Part model, mm, in its own coordinate system. Face numbers are marked on the shaded views. A direction names the side the tool comes from. Give positions to 0.01 mm unless a question says otherwise; leave off trailing zeros. Order: outer loops, then holes, each group sorted by start corner. A loop starts at its lowest first (then second) coordinate and runs counter-clockwise, first axis right, second up. Notation, with made-up numbers: (12.25, -10) - (46.25, -10) arc R12 ccw to (46.25, 13) - close; hole circle Ø9 at (-28, -36). An arc over 180 degrees is marked (long way). One line per item, written item: value.
```python
from build123d import *

# Parameters (mm, degrees)
SKETCH1_R                = 19
BOSS_EXTRUDE1_DEPTH      = 3.5
SKETCH2_R                = 30
SKETCH2_R_2              = 19
SKETCH2_R_3              = 2.8
BOSS_EXTRUDE2_DEPTH      = 7
BOSS_EXTRUDE3_DEPTH      = 2
BOSS_EXTRUDE3_DEPTH_BACK = 7
SKETCH4_R                = 2.9
SKETCH5_R                = 5
BOSS_EXTRUDE4_DEPTH      = 3
CUT_EXTRUDE1_START       = -10
SKETCH3_R                = 19
CUT_EXTRUDE1_DEPTH       = 10
CUT_EXTRUDE3_START       = -13
CUT_EXTRUDE3_DEPTH       = 13
FILLET1_R                = 10
FILLET2_R                = 5
CUT_EXTRUDE4_START       = -4
SKETCH8_R                = 4
SKETCH8_R_2              = 19
CUT_EXTRUDE4_DEPTH       = 4
FILLET3_R                = 1


with BuildPart() as part:
    # Sketch1 → Boss-Extrude1 (new body)
    with BuildSketch(Plane(origin=(0, 0, 0), x_dir=(1, 0, 0), z_dir=(0, 1, 0))):
        with Locations(Location((0, 0, 0), (0, 0, 270))):
            Circle(SKETCH1_R)
    extrude(amount=BOSS_EXTRUDE1_DEPTH)

    # Sketch2 → Boss-Extrude2 (add)
    with BuildSketch(Plane(origin=(0, 0, 0), x_dir=(1, 0, 0), z_dir=(0, 1, 0))):
        with Locations(Location((0, 0, 0), (0, 0, 270))):
            Circle(SKETCH2_R)
        with Locations(Location((0, 0, 0), (0, 0, 270))):
            Circle(SKETCH2_R_2, mode=Mode.SUBTRACT)
        with Locations(Location((0, 25, 0), (0, 0, 270))):
            Circle(SKETCH2_R_3, mode=Mode.SUBTRACT)
        with Locations(Location((21.650635095, -12.5, 0), (0, 0, 270))):
            Circle(SKETCH2_R_3, mode=Mode.SUBTRACT)
        with Locations(Location((-21.650635095, -12.5, 0), (0, 0, 270))):
            Circle(SKETCH2_R_3, mode=Mode.SUBTRACT)
    extrude(amount=BOSS_EXTRUDE2_DEPTH)

    # Sketch4 → Boss-Extrude3 (add, two sides: drawn at the far end of the back side and taken through both)
    with BuildSketch(Plane.XZ.offset(-BOSS_EXTRUDE3_DEPTH_BACK)):
        with Locations(Location((-21.650635095, 12.5, 0), (0, 0, 270))):
            Circle(SKETCH4_R)
        with Locations(Location((21.650635095, 12.5, 0), (0, 0, 270))):
            Circle(SKETCH4_R)
        with Locations(Location((0, -25, 0), (0, 0, 270))):
            Circle(SKETCH4_R)
    extrude(amount=BOSS_EXTRUDE3_DEPTH + BOSS_EXTRUDE3_DEPTH_BACK)

    # Sketch5 → Boss-Extrude4 (add)
    with BuildSketch(Plane(origin=(0, 7, 0), x_dir=(1, 0, 0), z_dir=(0, 1, 0))):
        with Locations((-26.103110985, -14.7860609)):
            Circle(SKETCH5_R)
        with Locations((0.246451131, 29.99898768)):
            Circle(SKETCH5_R)
        with Locations((25.856659853, -15.212926781)):
            Circle(SKETCH5_R)
    extrude(amount=-BOSS_EXTRUDE4_DEPTH)

    # Sketch3 → Cut-Extrude1 (cut)
    with BuildSketch(Plane(origin=(0, 3.5, 0), x_dir=(1, 0, 0), z_dir=(0, 1, 0)).offset(CUT_EXTRUDE1_START)):
        with Locations(Location((0, 0, 0), (0, 0, 270))):
            Circle(SKETCH3_R)
    extrude(amount=CUT_EXTRUDE1_DEPTH, mode=Mode.SUBTRACT)

    # Sketch7 → Cut-Extrude3 (cut)
    with BuildSketch(Plane(origin=(0, 7, 0), x_dir=(1, 0, 0), z_dir=(0, 1, 0)).offset(CUT_EXTRUDE3_START)):
        with BuildLine():
            ThreePointArc((-29.54423259, -5.20944533), (-25.980762114, 15), (-10.2606043, 28.190778624))
            Line((-10.2606043, 28.190778624), (-13.773984089, 37.84371026))
            Line((-13.773984089, 37.84371026), (-43.939319858, -7.747687605))
            Line((-43.939319858, -7.747687605), (-29.54423259, -5.20944533))
        make_face()
        with BuildLine():
            ThreePointArc((-26.13264562, -4.6078905), (-22.980662881, 13.267891901), (-9.075772579, 24.935480225))
            Line((-9.075772579, 24.935480225), (-10.2606043, 28.190778624))
            ThreePointArc((-10.2606043, 28.190778624), (-25.980762114, 15), (-29.54423259, -5.20944533))
            Line((-29.54423259, -5.20944533), (-26.13264562, -4.6078905))
        make_face()
        with BuildLine():
            Line((15.259965643, 41.926411025), (10.2606043, 28.190778624))
            ThreePointArc((10.2606043, 28.190778624), (25.980762114, 15), (29.54423259, -5.20944533))
            Line((29.54423259, -5.20944533), (39.660606503, -6.993234998))
            Line((39.660606503, -6.993234998), (15.259965643, 41.926411025))
        make_face()
        with BuildLine():
            Line((10.2606043, 28.190778624), (9.075772579, 24.935480225))
            ThreePointArc((9.075772579, 24.935480225), (21.736841548, 15.220300308), (26.535783801, 0))
            ThreePointArc((26.535783801, 0), (26.434807132, -2.312745947), (26.13264562, -4.6078905))
            Line((26.13264562, -4.6078905), (29.54423259, -5.20944533))
            ThreePointArc((29.54423259, -5.20944533), (25.980762114, 15), (10.2606043, 28.190778624))
        make_face()
        with BuildLine():
            Line((28.679354216, -34.17872342), (19.283628291, -22.981333294))
            ThreePointArc((19.283628291, -22.981333294), (0, -30), (-19.283628291, -22.981333294))
            Line((-19.283628291, -22.981333294), (-25.886622414, -30.850475262))
            Line((-25.886622414, -30.850475262), (28.679354216, -34.17872342))
        make_face()
        with BuildLine():
            Line((19.283628291, -22.981333294), (17.056873041, -20.327589725))
            ThreePointArc((17.056873041, -20.327589725), (0, -26.535783801), (-17.056873041, -20.327589725))
            Line((-17.056873041, -20.327589725), (-19.283628291, -22.981333294))
            ThreePointArc((-19.283628291, -22.981333294), (0, -30), (19.283628291, -22.981333294))
        make_face()
    extrude(amount=CUT_EXTRUDE3_DEPTH, mode=Mode.SUBTRACT)

    # Fillet1
    # the kernel refuses this fillet: 10 mm, written as the material it adds along each edge
    with BuildSketch(Plane(origin=(-26.13264562, 0, 4.6078905), x_dir=(-0.9848077530122318, 0, 0.17364817766679624), z_dir=(0, 1, 0)), Plane(origin=(17.056873041, 0, 20.327589725), x_dir=(0.6427876096865569, 0, 0.7660444431189634), z_dir=(0, 1, 0)), Plane(origin=(9.075772579, 0, -24.935480225), x_dir=(0.34202014332561265, 0, -0.9396926207859289), z_dir=(0, 1, 0))) as fillet1_piece_1:
        with BuildLine():
            CenterArc((9.045274498, -8.297697769), FILLET1_R, 123.92490422, 42.948020906)
            Line((-0.693413056, -6.026582466), (-0.888186807, -5.98116016))
            ThreePointArc((-0.888186807, -5.98116016), (-0.372612378, -3.01031053), (-0.2, 0))
            Line((-0.2, 0), (0, 0.2))
            ThreePointArc((0, 0.2), (1.732108099, 0.2), (3.352595033, 0.165953955))
            Line((3.352595033, 0.165953955), (3.464216199, 0))
        make_face()
    extrude(amount=7)
    with BuildSketch(Plane(origin=(-17.056873041, 0, 20.327589725), x_dir=(0.8344973728156843, 0, 0.551011918894429), z_dir=(0, 1, 0)), Plane(origin=(26.13264562, 0, 4.6078905), x_dir=(0.059941633142754296, 0, -0.99820188369697), z_dir=(0, 1, 0)), Plane(origin=(-9.075772579, 0, -24.935480225), x_dir=(-0.8944390059584274, 0, 0.44718996480254386), z_dir=(0, 1, 0))) as fillet1_piece_2:
        with BuildLine():
            CenterArc((7.20939257, -9.934457095), FILLET1_R, 96.563537437, 42.948020906)
            Line((-0.39597707, -3.441510719), (-0.548084463, -3.311651792))
            ThreePointArc((-0.548084463, -3.311651792), (-0.396677677, -1.697894369), (-0.198689142, 0.022860991))
            Line((-0.198689142, 0.022860991), (0.022860991, 0.198689142))
            ThreePointArc((0.022860991, 0.198689142), (3.03317152, 0.026076764), (6.04348205, 0.198689142))
            Line((6.04348205, 0.198689142), (6.06634304, 0))
        make_face()
    extrude(amount=7)

    # Fillet2
    fillet2_edges = [part.edges().sort_by_distance(p)[0] for p in [
        (-10.2606043, 3.5, -28.190778624),
        (-29.54423259, 3.5, 5.20944533),
        (-19.283628291, 3.5, 22.981333294),
        (19.283628291, 3.5, 22.981333294),
        (29.54423259, 3.5, 5.20944533),
        (10.2606043, 3.5, -28.190778624),
    ]]
    fillet(fillet2_edges, radius=FILLET2_R)

    # Sketch8 → Cut-Extrude4 (cut)
    with BuildSketch(Plane(origin=(0, 7, 0), x_dir=(1, 0, 0), z_dir=(0, 1, 0)).offset(CUT_EXTRUDE4_START)):
        with Locations((-16.524893724, 9.376987118)):
            Circle(SKETCH8_R)
        with Locations(Location((0, 0, 0), (0, 0, 42.512080704))):
            Circle(SKETCH8_R_2)
        with Locations((16.383155917, 9.622484201)):
            Circle(SKETCH8_R)
        with Locations((0.141737807, -18.999471319)):
            Circle(SKETCH8_R)
    extrude(amount=CUT_EXTRUDE4_DEPTH, mode=Mode.SUBTRACT)

    # Fillet3
    # the kernel refuses this fillet: 1 mm, written as the material it takes off along each edge
    with BuildSketch(Plane(origin=(-14.195555863, 8.950278825, -12.628784333), x_dir=(-0.8617980531882996, 0, -0.5072515308216002), z_dir=(0, -1, 0)), Plane(origin=(18.034625983, 8.950278825, -5.979319831), x_dir=(0.8701917383942803, 0, -0.49271324158209956), z_dir=(0, -1, 0))) as fillet3_piece_1:
        with BuildLine():
            CenterArc((0.805364366, 0.995988176), FILLET3_R, 193.528948716, 71.337075115)
            ThreePointArc((-0.166887482, 0.762051552), (-0.079532242, 0.381882385), (0, 0))
            ThreePointArc((0, 0), (0.357939718, 0.016047295), (0.715879437, 0))
        make_face()
    extrude(amount=5.950278825, mode=Mode.SUBTRACT)
    with BuildSketch(Plane(origin=(-18.121826323, 8.950278825, -5.709589366), x_dir=(-0.28086097725665193, 0, 0.9597484625955065), z_dir=(0, -1, 0)), Plane(origin=(14.005562597, 8.950278825, -12.839167276), x_dir=(-0.6907360612225409, 0, -0.7231069725336425), z_dir=(0, -1, 0))) as fillet3_piece_2:
        with BuildLine():
            CenterArc((0.800640781, 0.999789253), FILLET3_R, 197.486602821, 71.337075115)
            ThreePointArc((-0.153146456, 0.699306464), (-0.060897436, 0.353086193), (0, 0))
            ThreePointArc((0, 0), (0.390055765, 0.004004198), (0.78011153, 0))
        make_face()
    extrude(amount=5.950278825, mode=Mode.SUBTRACT)
    with BuildSketch(Plane(origin=(-3.83907012, 8.950278825, 18.608104165), x_dir=(-0.9750194381231715, 0, -0.22211955177780904), z_dir=(0, -1, 0))) as fillet3_piece_3:
        with BuildLine():
            CenterArc((0.800640781, -0.999789253), FILLET3_R, 91.176322064, 71.337075115)
            ThreePointArc((-0.153146456, -0.699306464), (-0.060897436, -0.353086193), (0, 0))
            ThreePointArc((0, 0), (0.390055765, -0.004004198), (0.78011153, 0))
        make_face()
    extrude(amount=5.950278825, mode=Mode.SUBTRACT)
    with BuildSketch(Plane(origin=(4.116263726, 8.950278825, 18.548756641), x_dir=(0.023311579398747933, 0, 0.9997282482084497), z_dir=(0, -1, 0))) as fillet3_piece_4:
        with BuildLine():
            CenterArc((0.805364366, -0.995988176), FILLET3_R, 95.133976169, 71.337075115)
            ThreePointArc((-0.166887482, -0.762051552), (-0.079532242, -0.381882385), (0, 0))
            ThreePointArc((0, 0), (0.357939718, -0.016047295), (0.715879437, 0))
        make_face()
    extrude(amount=5.950278825, mode=Mode.SUBTRACT)


solid = part.part
```
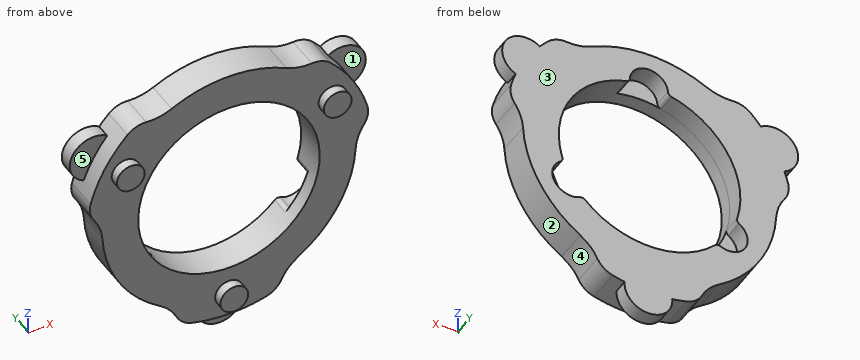
1) Which spindle directions (+Z, -Z, +X, -X, +Y, -Y) get a long thin tool onto all of the face, cutting with end or side? Do the marked faces 4 and 5. Say none if no direction does.
Answer:
face 4: -Z, +X, +Y, -Y
face 5: +Z, -X, -Y
2) Two-plate mould, pull along Y, no slides. Class the marked faces 1, 2 and 3: pulls with the +Y half, pulls with the -Y half, needs draft (parallel to the pull), parting line crosses it, or undercut.
Answer:
face 1: pulls with the -Y half
face 2: needs draft
face 3: pulls with the +Y half
3) Wall check: line 1 along Z through (x, y) = (0, 3.5); line 2 along Z through (x, y) = (0, 2.5); line 3 along Y through (x, z) = (-26.5, 6). Give the ranges that are in metal, low to high. Write a range as [from, to].
Answer:
line 1: z = [-30, -19], [23, 26.54]
line 2: z = [-30, -19], [19, 26.54]
line 3: y = [0, 7]
4) Slice it at A-A on z = 0. Write the cut outline in (x, y).
Answer:
outline: (-26.68, 0) - (-19, 0) - (-19, 7) - (-26.68, 7) - close; (19, 0) - (26.68, 0) - (26.68, 7) - (19, 7) - close
5) Drop flat-ended pins along their axis: P1, Ø1, axis at x = 21, y = 1.5, coming from the +Z side; P2, Ø2, axis at x = -17.5, z = -9.5, coming from the +Y side; P3, Ø4, axis at x = 11.5, y = -0.5, coming from the -Z side. Give the stop position or say it passes through.
Answer:
P1: stops at z = 21.79
P2: stops at y = 3
P3: stops at z = -28.05
6) Slice it at B-B on x = -6.5. Write the cut outline in (y, z), then the cut area to 3 significant figures.
Answer:
outline: (0, -29.29) - (7, -29.29) - (7, -17.85) - (0, -17.85) - close; (0, 17.85) - (7, 17.85) - (7, 25.73) - (0, 25.73) - close
area: 135 mm2
7) Slice it at D-D on x = 0. Write the cut outline in (y, z).
Answer:
outline: (-2, -27.9) - (0, -27.9) - (0, -30) - (4, -30) - (4, -34.99) - (7, -34.99) - (7, -19) - (0, -19) - (0, -22.1) - (-2, -22.1) - close; (0, 19) - (3, 19) - (3, 23) - (7, 23) - (7, 26.54) - (0, 26.54) - close
8) Slice it at C-C on z = -25. Write the cut outline in (x, y).
Answer:
outline: (-11.68, 0) - (-2.9, 0) - (-2.9, -2) - (2.9, -2) - (2.9, 0) - (11.68, 0) - (11.68, 7) - (-11.68, 7) - close
